from build123d import *

# Parameters (mm, degrees)
F2_SIZE  = 2
F5_DEPTH = 5
F6_DEPTH = 10


with BuildPart() as f1:
    # F0 (on Top) → F1 (revolve)
    with BuildSketch(Plane.XY):
        Polygon((-22.5, 0), (0, 0), (0, 166.7), (-20, 166.7), (-20, 116.7), (-22.5, 116.7), (-22.5, 76.7), (-28.5, 76.7), (-28.5, 68), (-25, 68), (-25, 28), (-22.5, 28), align=None)
    revolve(axis=Axis((0, 59.789897, 0), (0, -1, 0)))

    # F2
    f2_edges = [f1.edges().sort_by_distance(p)[0] for p in [
        (20, 166.7, 0),
        (22.5, 0, 0),
    ]]
    chamfer(f2_edges, length=F2_SIZE)

    # F4 (on offset) → F5 (cut)
    with BuildSketch(Plane.XY.offset(25)):
        with BuildLine():
            Line((7, 40), (7, 56))
            ThreePointArc((7, 56), (4.949747, 60.949747), (0, 63))
            ThreePointArc((0, 63), (-4.949747, 60.949747), (-7, 56))
            Line((-7, 56), (-7, 40))
            ThreePointArc((-7, 40), (-4.949747, 35.050253), (0, 33))
            ThreePointArc((0, 33), (4.949747, 35.050253), (7, 40))
        make_face()
    extrude(amount=-F5_DEPTH, mode=Mode.SUBTRACT)

    # F4 (on offset) → F6 (cut)
    with BuildSketch(Plane.XY.offset(25)):
        with BuildLine():
            Line((7, 133.7), (7, 149.7))
            ThreePointArc((7, 149.7), (4.949747, 154.649747), (0, 156.7))
            ThreePointArc((0, 156.7), (-4.949747, 154.649747), (-7, 149.7))
            Line((-7, 149.7), (-7, 133.7))
            ThreePointArc((-7, 133.7), (-4.949747, 128.750253), (0, 126.7))
            ThreePointArc((0, 126.7), (4.949747, 128.750253), (7, 133.7))
        make_face()
    extrude(amount=-F6_DEPTH, mode=Mode.SUBTRACT)


solid = f1.part
Design review of the part built by this model. Coordinates are the model's own, in mm. A direction names the side the tool comes from. Coordinates: 2 decimals unless noted, no trailing zeros. Order: outer loops, then holes, each group sorted by start corner. A loop starts at its lowest first (then second) coordinate and runs counter-clockwise, first axis right, second up.
Item 1: Take a section at A-A, the plane z = 0. Write out the cut boundary in (x, y), then the cut area to 3 significant figures.
Item 2: For line 1 (Y direction, x = -20, z = 13.5); line 2 (Z direction, x = -0.5, y = 126.5); line 3 (Y direction, x = -4, z = -26), list the stretches that pass through material, from the lowest coordinate up.
Item 3: For faces 5 (the flat face through (0.1, 68, 25.2)), 6 (the cylindrical face through (-10.382, 96.42, 19.961)), 7 (the flat face through (-7, 48, 22)), list the 3-axis set-ups (+Z, -Z, +X, -X, +Y, -Y) from which the entire face can be reached by the end or side of a thin tool; tool diameter is ignored.
Item 4: Take a section at C-C, the plane y = 84.5. Write out the cut boundary in (x, z), then the cut area to 3 significant figures.
Item 5: For pin 1 Ø2 at (x, y) = (9.5, 27.5) entering from +Z; pin 2 Ø1.5 at (x, y) = (11, 57.5) entering from -Z; pin 3 Ø8 at (y, z) = (115, -1.5) entering from -X, all flat-tipped, find the tip position at first contact; note any pin that passes through.
Item 6: Take a section at B-B, the plane y = 122.5. Write out the cut boundary in (x, z).
Item 7: The part is to be moulded in two halves that separate along X. For faces 1 (the flat face through (0, 48, 20)), 2 (the conical face through (-17.288, 166.575, -5.444)), 3 (the flat face through (-20.1, 116.7, 1.6)), 4 (the flat face through (7, 142, 17)), say which applies: pulls with the +X half, pulls with the -X half, needs draft (parallel to the pull), parting line crosses it, or undercut.
Item 8: Take a section at D-D, the plane y = 43.5. Write out the cut boundary in (x, z).
The answers:
1. outline: (-28.5, 68) - (-25, 68) - (-25, 28) - (-22.5, 28) - (-22.5, 2) - (-20.5, 0) - (20.5, 0) - (22.5, 2) - (22.5, 28) - (25, 28) - (25, 68) - (28.5, 68) - (28.5, 76.7) - (22.5, 76.7) - (22.5, 116.7) - (20, 116.7) - (20, 164.7) - (18, 166.7) - (-18, 166.7) - (-20, 164.7) - (-20, 116.7) - (-22.5, 116.7) - (-22.5, 76.7) - (-28.5, 76.7) - close
1. area: 7,550 mm2
2. line 1: y = 28 to 76.7
2. line 2: z = -19.99 to 19.99
2. line 3: y = 68 to 76.7
3. face 5: -Y
3. face 6: +Y
3. face 7: +Z
4. outline: circle Ø45 at (0, 0)
4. area: 1,590 mm2
5. pin 1: stops at z = 23.46
5. pin 2: stops at z = -22.8
5. pin 3: stops at x = -22.5
6. outline: circle Ø40 at (0, 0)
7. face 1: undercut
7. face 2: parting line crosses it
7. face 3: needs draft
7. face 4: undercut
8. outline: (-7, 20) - (-7, 24) arc R25 ccw (long way) to (7, 24) - (7, 20) - close
